Work out the finished part from the listing and answer in its coordinate system (mm). A direction names the side the tool comes from. Round coordinates to 2 decimals unless told otherwise and drop trailing zeros. Write each loop counter-clockwise with the first axis right and the second up, starting at its lowest first coordinate (ties: lowest second). Pieces come first, ordered by that corner, then holes. Notation, with made-up numbers: (15.5, -8) -> (62.5, -8) arc R22 cw to (62.5, 7) -> close; hole circle Ø10 at (42.25, -16). An arc over 180 degrees is marked (long way). One line per item, written item: value.
```python
from build123d import *

# Parameters (mm, degrees)
SKETCH_1_W          = 27.8
SKETCH_1_H          = 8
EXTRUDE_1_DEPTH     = 7.8
EXTRUDE_2_DEPTH     = 27.8
SKETCH_4_R          = 1.15
EXTRUDE_3_DEPTH     = 2
CUT_EXTRUDE_4_DEPTH = 24.8
SKETCH_15_W         = 27.8
SKETCH_15_H         = 4.251772847
EXTRUDE_4_DEPTH     = 1.9
FILLET_1_R          = 8
FILLET_2_R          = 9.5
EXTRUDE_5_DEPTH     = 27.8
CUT_EXTRUDE_6_DEPTH = 24.8
CUT_EXTRUDE_7_DEPTH = 40.8
SKETCH_21_W         = 2.6
SKETCH_21_H         = 3
EXTRUDE_6_DEPTH     = 1
CUT_EXTRUDE_8_DEPTH = 3
CUT_EXTRUDE_9_DEPTH = 0.5


with BuildPart() as part:
    # 草图1 → 凸台-拉伸1 (new body)
    with BuildSketch(Plane.XY):
        with Locations((13.9, -4)):
            Rectangle(SKETCH_1_W, SKETCH_1_H)
    extrude(amount=EXTRUDE_1_DEPTH)

    # 草图2 → 凸台-拉伸2 (add)
    with BuildSketch(Plane.ZY):
        Polygon((5.795554958, -15.947085729), (0, -17.5), (0, -8), (7.8, -8), align=None)
    extrude(amount=-EXTRUDE_2_DEPTH)

    # 草图4 → 凸台-拉伸3 (add)
    with BuildSketch(Plane(origin=(0, 0, -1.9), x_dir=(-1, 0, 0), z_dir=(0, 0, -1))):
        with BuildLine():
            Line((0, -2), (0, -4.7))
            Line((0, -4.7), (6, -4.7))
            ThreePointArc((6, -4.7), (6.353553391, -4.553553391), (6.5, -4.2))
            Line((6.5, -4.2), (6.5, -2))
            Line((6.5, -2), (6.5, 2.4))
            ThreePointArc((6.5, 2.4), (6.353553391, 2.753553391), (6, 2.9))
            Line((6, 2.9), (4, 2.9))
            ThreePointArc((4, 2.9), (2.232233047, 2.167766953), (1.5, 0.4))
            Line((1.5, 0.4), (1.5, -1.5))
            ThreePointArc((1.5, -1.5), (1.353553391, -1.853553391), (1, -2))
            Line((1, -2), (0, -2))
        make_face()
        with Locations((3.6, 0.5)):
            Circle(SKETCH_4_R, mode=Mode.SUBTRACT)
    extrude_3 = extrude(amount=-EXTRUDE_3_DEPTH)

    # 镜向1: 凸台-拉伸3 across plane
    add(extrude_3.mirror(Plane.ZY.offset(-13.9)))

    # 草图13 → 切除-拉伸4 (cut)
    with BuildSketch(Plane.ZY.offset(-1.5)):
        Polygon((1.5, 0), (1.5, -11.921695309), (0, -12.323619098), (0, -15.947085729), (4.556522218, -14.726169281), (6.3, -7.813748582), (6.3, 0), align=None)
    extrude(amount=-CUT_EXTRUDE_4_DEPTH, mode=Mode.SUBTRACT)

    # 草图15 → 凸台-拉伸4 (add)
    with BuildSketch(Plane(origin=(0, 0, 0), x_dir=(-1, 0, 0), z_dir=(0, 0, -1))):
        with Locations((-13.9, -4.125886424)):
            Rectangle(SKETCH_15_W, SKETCH_15_H)
    extrude(amount=EXTRUDE_4_DEPTH)

    # 圆角1
    fillet_1_edges = [part.edges().sort_by_distance(p)[0] for p in [
        (13.9, -14.726169281, 4.556522218),
    ]]
    fillet(fillet_1_edges, radius=FILLET_1_R)

    # 圆角2
    fillet_2_edges = [part.edges().sort_by_distance(p)[0] for p in [
        (13.9, -15.947085729, 5.795554958),
    ]]
    fillet(fillet_2_edges, radius=FILLET_2_R)

    # 草图17 → 凸台-拉伸5 (add)
    with BuildSketch(Plane(origin=(27.8, 0, 0), x_dir=(0, 0, -1), z_dir=(1, 0, 0))):
        Polygon((0, -17.5), (7, -19.375644347), (7, -12.646349174), (0, -10.770704827), align=None)
    extrude(amount=-EXTRUDE_5_DEPTH)

    # 草图18 → 切除-拉伸6 (cut)
    with BuildSketch(Plane.ZY.offset(-26.3)):
        Polygon((0, -12.323619098), (0, -15.947085729), (-7, -17.822730076), (-7, -14.199263445), align=None)
    extrude(amount=CUT_EXTRUDE_6_DEPTH, mode=Mode.SUBTRACT)

    # 草图19 → 切除-拉伸7 (cut)
    with BuildSketch(Plane(origin=(34.3, 0, 0), x_dir=(0, 0, -1), z_dir=(1, 0, 0))):
        Polygon((7, 2.9), (7, -14.199263445), (-1.5, -11.921695309), (-1.5, 2.9), align=None)
    extrude(amount=-CUT_EXTRUDE_7_DEPTH, mode=Mode.SUBTRACT)

    # 草图21 → 凸台-拉伸6 (add)
    with BuildSketch(Plane.ZY):
        with Locations((3.3, -7.99)):
            Rectangle(SKETCH_21_W, SKETCH_21_H)
    extrude_6 = extrude(amount=EXTRUDE_6_DEPTH)

    # 草图22 → 切除-拉伸8 (cut)
    with BuildSketch(Plane(origin=(0, -9.49, 0), x_dir=(-1, 0, 0), z_dir=(0, -1, 0))):
        Polygon((0, -2), (1, -4.1), (1, -2), align=None)
    cut_extrude_8 = extrude(amount=-CUT_EXTRUDE_8_DEPTH, mode=Mode.SUBTRACT)

    # 镜向5: 凸台-拉伸6, 切除-拉伸8 across plane
    add(extrude_6.mirror(Plane.ZY.offset(-13.9)))
    add(cut_extrude_8.mirror(Plane.ZY.offset(-13.9)), mode=Mode.SUBTRACT)

    # 草图23 → 切除-拉伸9 (cut)
    with BuildSketch(Plane.ZY.offset(-26.3)):
        Polygon((2.3, -12.5355569), (-7, -15.027484389), (-7, -14.199263445), (1.5, -11.921695309), (1.5, 0), (2.3, 0), align=None)
    cut_extrude_9 = extrude(amount=-CUT_EXTRUDE_9_DEPTH, mode=Mode.SUBTRACT)

    # 镜向6: 切除-拉伸9 across plane
    add(cut_extrude_9.mirror(Plane.ZY.offset(-13.9)), mode=Mode.SUBTRACT)


solid = part.part
```
(1) Find section B-B on x = 17.5. Give the vertices of the cut face in (y, z).
Reported:
outline: (-19.38, -7) -> (-17.82, -7) -> (-15.94, 0.02) arc R8 cw to (-10.17, 5.71) -> (-7.81, 6.3) -> (0, 6.3) -> (0, 7.8) -> (-8, 7.8) -> (-10.54, 7.16) arc R9.5 ccw to (-17.39, 0.41) -> close
(2) Consider probe 1 along X at (y, z) = (-13, 1.5); probe 2 along Z at (x, y) = (20.75, -3.25); probe 3 along Z at (x, y) = (26.5, -3). Determine where each line is inside the solid, lowest interval first.
Reported:
probe 1: x = 0 to 1.5, 26.3 to 27.8
probe 2: z = 6.3 to 7.8
probe 3: z = 2.3 to 7.8
(3) Find section C-C on z = 3.5. Give the vertices of the cut face in (x, y), plus the area to 3 significant figures.
Reported:
outline: (-0.71, -9.49) -> (0, -9.49) -> (0, -15.92) -> (27.8, -15.92) -> (27.8, -9.49) -> (28.51, -9.49) -> (28.51, -6.49) -> (27.8, -6.49) -> (27.8, 0) -> (26.3, 0) -> (26.3, -13.97) -> (1.5, -13.97) -> (1.5, 0) -> (0, 0) -> (0, -6.49) -> (-0.71, -6.49) -> close
area: 100 mm2
(4) Flat-ended cylindrical pins translate along their axes: pin 1 Ø4.5 at (y, z) = (-12, 0) entering from -X; pin 2 Ø1.1 at (x, y) = (-0.5, -8) entering from +Z; pin 3 Ø1 at (y, z) = (-2.5, 0.5) entering from +X; pin 4 Ø6.5 at (x, y) = (9, -5.5) entering from -Z. Find the tip coordinate at first contact, or state that the pin passes through.
Reported:
pin 1: stops at x = 0
pin 2: stops at z = 7.8
pin 3: passes through
pin 4: stops at z = 6.06
(5) A tool of negligible diameter and unlimited length cuts with its end or side. For faces 1 (the face through (1, -10, 2)), 2 (the face through (-0.4, -6.49, 3.6)), 3 (the face through (28, -6.49, 4)), from which of +Z, -Z, +X, -X, +Y, -Y can it reach the whole face along a straight path? Write none if from no direction.
Reported:
face 1: -Z, +Y
face 2: +Z, -Z, -X, +Y
face 3: +Z, -Z, +X, +Y
(6) For a pull along X with two mould halves and no side action, classify faces 4 (the face through (26.8, -10, 2)), 5 (the face through (17, -18, -7)), 6 (the face through (-0.493, -8.011, 3.035)) as pulls with the +X half, pulls with the -X half, needs draft (parallel to the pull), parting line crosses it, or undercut.
Reported:
face 4: undercut
face 5: needs draft
face 6: pulls with the -X half
(7) Find section D-D on y = -16.75. Give the vertices of the cut face in (x, z).
Reported:
outline: (0, -7) -> (1.5, -7) -> (1.5, -3) -> (26.3, -3) -> (26.3, -7) -> (27.8, -7) -> (27.8, 2.12) -> (0, 2.12) -> close
(8) Find section A-A on y = -4.75. Give the vertices of the cut face in (x, z).
Reported:
outline: (0, 1.5) -> (1, 1.5) -> (1, 2.3) -> (1.5, 2.3) -> (1.5, 6.3) -> (26.3, 6.3) -> (26.3, 2.3) -> (26.8, 2.3) -> (26.8, 1.5) -> (27.8, 1.5) -> (27.8, 7.8) -> (0, 7.8) -> close
